Part print with two shaded views. Sizes in mm from the minimum x, y, z corner. Round coordinates to 2 decimals unless told otherwise and drop trailing zeros. Order: outer loops, then holes, each group sorted by start corner. A loop starts at its lowest first (then second) coordinate and runs counter-clockwise, first axis right, second up. Notation, with made-up numbers: M -32,-0.5 L -26,-0.5 A15 ccw -26,17.5 Z; hole C 11,85.5 d1. An arc over 180 degrees is marked long. One line per question, with ' | ' between items.
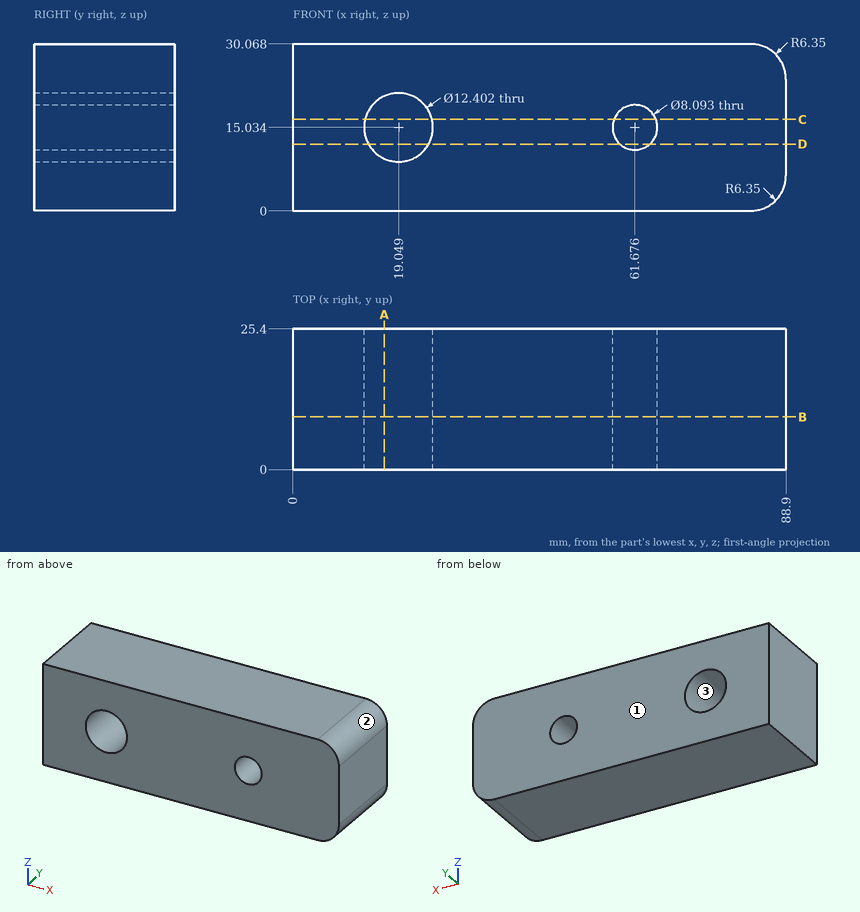
1) Drop flat-ended pins along their axis: pin 1 (3 mm diameter, centred on y = 18.5, z = 4, fed in from +X); pin 2 (1.5 mm diameter, centred on x = 68.5, z = 23, fed in from -Y). Give the stop position or say it passes through.
The answers:
pin 1: stops at x = 88.84 | pin 2: stops at y = 0
2) Saw through at B-B (y = 9.5). Give the number of separate pieces and of enclosed holes in the cut face, plus the area to 3 significant figures.
The answers:
separate pieces: 1 | enclosed holes: 2 | area: 2,480 mm²
3) Saw through at A-A (x = 16.5). List the corners of the cut face in (y, z).
The answers:
outline: M 0,0 L 25.4,0 L 25.4,9.38 L 0,9.38 Z; M 0,20.69 L 25.4,20.69 L 25.4,30.07 L 0,30.07 Z
4) Saw through at C-C (z = 16.5). List the corners of the cut face in (x, y) (1 decimal).
The answers:
outline: M 0,0 L 13,0 L 13,25.4 L 0,25.4 Z; M 25.1,0 L 57.9,0 L 57.9,25.4 L 25.1,25.4 Z; M 65.4,0 L 88.9,0 L 88.9,25.4 L 65.4,25.4 Z
5) Saw through at D-D (z = 12). List the corners of the cut face in (x, y).
The answers:
outline: M 0,0 L 13.64,0 L 13.64,25.4 L 0,25.4 Z; M 24.46,0 L 59,0 L 59,25.4 L 24.46,25.4 Z; M 64.35,0 L 88.9,0 L 88.9,25.4 L 64.35,25.4 Z
6) Probe line 1 (X direction, y = 15.5, z = 15); line 2 (X direction, y = 20.25, z = 15.5) (1 decimal); line 3 (Z direction, x = 61, y = 9.5) (1 decimal). List the from-to ranges inside material, lowest first. Write a range as [from, to].
The answers:
line 1: x = [0, 12.85], [25.25, 57.63], [65.72, 88.9] | line 2: x = [0, 12.9], [25.2, 57.7], [65.7, 88.9] | line 3: z = [0, 11], [19, 30.1]
7) Two-plate mould, pull along X, no slides. Class the marked faces 1, 2 and 3: released by +X, released by -X, zero draft, split by the parting line, or undercut.
The answers:
face 1: zero draft | face 2: released by +X | face 3: undercut
